Read the model definition and answer for the solid it produces. Units are mm, in the model's axes. Coordinates: 2 decimals unless noted, no trailing zeros. Loops run counter-clockwise (first coordinate to the right, second up) from the corner with the lowest first, then second, coordinate; pieces in that order, holes last.
from build123d import *

# Parameters (mm, degrees)
SKETCH1_R           = 0.75
BOSS_EXTRUDE1_DEPTH = 50
FILLET1_R           = 0.75


with BuildPart() as part:
    # Sketch1 → Boss-Extrude1 (new body)
    with BuildSketch(Plane.XY):
        Circle(SKETCH1_R)
    extrude(amount=BOSS_EXTRUDE1_DEPTH)

    # Sketch2 → Revolve1 (revolve)
    with BuildSketch(Plane.XY.offset(50)):
        with BuildLine():
            Line((-1, 0), (1, 0))
            ThreePointArc((1, 0), (0, 1), (-1, 0))
        make_face()
    revolve(axis=Axis((-1, 0, 50), (1, 0, 0)))

    # Fillet1
    fillet1_edges = [part.edges().sort_by_distance(p)[0] for p in [
        (-0.75, 0, 0),
    ]]
    fillet(fillet1_edges, radius=FILLET1_R)


solid = part.part
Q1. A cutting plane is placed at B-B (y = 0). Give the vertices of the cut face in (x, z).
Findings below:
outline: (-0.75, 0.75) arc R0.75 ccw to (0.75, 0.75) - (0.75, 49.34) arc R1 ccw (long way) to (-0.75, 49.34) - close
Q2. Straight lines are drawn through the part: probe 1 along X at (y, z) = (0.1, 42.5); probe 2 along Y at (x, z) = (-0.05, 9); probe 3 along Z at (x, y) = (-0.2, -0.8). For each, find the intervals that lie inside material, in ascending order.
Findings below:
probe 1: x = -0.74 to 0.74
probe 2: y = -0.75 to 0.75
probe 3: z = 49.43 to 50.57
Q3. A cutting plane is placed at C-C (x = 0.45). Give the vertices of the cut face in (y, z), then the cut area to 3 significant figures.
Findings below:
outline: (-0.6, 0.75) arc R0.6 ccw to (0.6, 0.75) - (0.6, 49.34) arc R0.89 ccw (long way) to (-0.6, 49.34) - close
area: 61.2 mm2
Q4. Flat-ended cylindrical pins translate along their axes: pin 1 Ø1 at (y, z) = (0.5, 25) entering from -X; pin 2 Ø1 at (x, z) = (0.5, 13.5) entering from -Y. Find the tip coordinate at first contact, or state that the pin passes through.
Findings below:
pin 1: stops at x = -0.75
pin 2: stops at y = -0.75
Q5. A cutting plane is placed at A-A (z = 40). Give the vertices of the cut face in (x, y).
Findings below:
outline: circle Ø1.5 at (0, 0)
